The listing builds one solid part. Answer for the finished solid, in the listing's coordinates (mm). Round coordinates to 2 decimals unless told otherwise and drop trailing zeros. Loops run counter-clockwise (first coordinate to the right, second up) from the corner with the lowest first, then second, coordinate; pieces in that order, holes last. Notation, with made-up numbers: (-1, 83.5) -> (21, 83.5) arc R15 cw to (21, 99.5) -> close; hole circle Ø10 at (-29.5, 75.25). An arc over 180 degrees is marked (long way). Write each question's results on one line, items separated by ' | '. Start each with the question number.
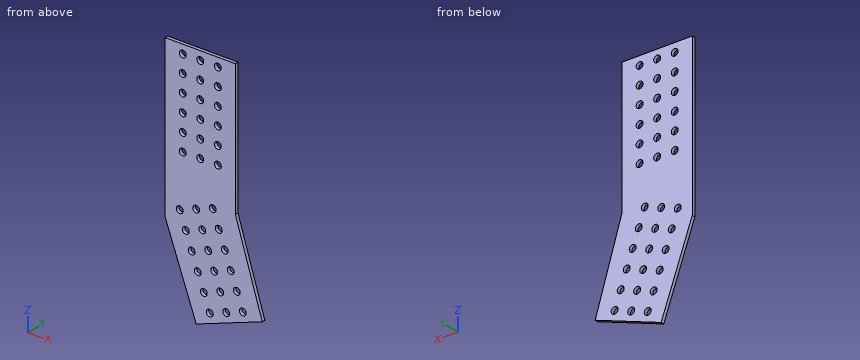
from build123d import *

# Parameters (mm, degrees)
SKETCH1_W           = 50.8
SKETCH1_H           = 76.2
SKETCH1_R           = 2.4892
BOSS_EXTRUDE1_DEPTH = 2.38125


with BuildPart() as part:
    # Sketch1 → Boss-Extrude1 (new body)
    # profile 1 of 3: a face of its own
    with BuildSketch(Plane(origin=(0, 0, 0), x_dir=(1, 0, 0), z_dir=(0, 1, 0))):
        with Locations((-99.145518613, -345.905622456)):
            Rectangle(SKETCH1_W, SKETCH1_H)
        with Locations(Location((-86.445518613, -326.855622456, 0), (0, 0, 90))):
            Circle(SKETCH1_R, mode=Mode.SUBTRACT)
        with Locations(Location((-86.445518613, -352.255622456, 0), (0, 0, 90))):
            Circle(SKETCH1_R, mode=Mode.SUBTRACT)
        with Locations(Location((-86.445518613, -377.655622456, 0), (0, 0, 90))):
            Circle(SKETCH1_R, mode=Mode.SUBTRACT)
        with Locations(Location((-99.145518613, -326.855622456, 0), (0, 0, 90))):
            Circle(SKETCH1_R, mode=Mode.SUBTRACT)
        with Locations(Location((-99.145518613, -352.255622456, 0), (0, 0, 90))):
            Circle(SKETCH1_R, mode=Mode.SUBTRACT)
        with Locations(Location((-99.145518613, -377.655622456, 0), (0, 0, 90))):
            Circle(SKETCH1_R, mode=Mode.SUBTRACT)
        with Locations(Location((-111.845518613, -377.655622456, 0), (0, 0, 90))):
            Circle(SKETCH1_R, mode=Mode.SUBTRACT)
        with Locations(Location((-111.845518613, -364.955622456, 0), (0, 0, 90))):
            Circle(SKETCH1_R, mode=Mode.SUBTRACT)
        with Locations(Location((-111.845518613, -352.255622456, 0), (0, 0, 90))):
            Circle(SKETCH1_R, mode=Mode.SUBTRACT)
        with Locations(Location((-111.845518613, -339.555622456, 0), (0, 0, 90))):
            Circle(SKETCH1_R, mode=Mode.SUBTRACT)
        with Locations(Location((-111.845518613, -326.855622456, 0), (0, 0, 90))):
            Circle(SKETCH1_R, mode=Mode.SUBTRACT)
        with Locations(Location((-111.845518613, -314.155622456, 0), (0, 0, 90))):
            Circle(SKETCH1_R, mode=Mode.SUBTRACT)
        with Locations(Location((-99.145518613, -364.955622456, 0), (0, 0, 90))):
            Circle(SKETCH1_R, mode=Mode.SUBTRACT)
        with Locations(Location((-99.145518613, -339.555622456, 0), (0, 0, 90))):
            Circle(SKETCH1_R, mode=Mode.SUBTRACT)
        with Locations(Location((-99.145518613, -314.155622456, 0), (0, 0, 90))):
            Circle(SKETCH1_R, mode=Mode.SUBTRACT)
        with Locations(Location((-86.445518613, -364.955622456, 0), (0, 0, 90))):
            Circle(SKETCH1_R, mode=Mode.SUBTRACT)
        with Locations(Location((-86.445518613, -339.555622456, 0), (0, 0, 90))):
            Circle(SKETCH1_R, mode=Mode.SUBTRACT)
        with Locations(Location((-86.445518613, -314.155622456, 0), (0, 0, 90))):
            Circle(SKETCH1_R, mode=Mode.SUBTRACT)
    # profile 2 of 3: a face of its own
    with BuildSketch(Plane(origin=(0, 0, 0), x_dir=(1, 0, 0), z_dir=(0, 1, 0))):
        Polygon((-73.745518613, -307.805622456), (-124.545518613, -307.805622456), (-124.545518613, -267.92136832), (-73.745518613, -286.411056221), align=None)
        with Locations(Location((-102.075911776, -280.451262674, 0), (0, 0, 90))):
            Circle(SKETCH1_R, mode=Mode.SUBTRACT)
        with Locations(Location((-114.01000806, -276.107606853, 0), (0, 0, 90))):
            Circle(SKETCH1_R, mode=Mode.SUBTRACT)
        with Locations(Location((-90.141815492, -284.794918494, 0), (0, 0, 90))):
            Circle(SKETCH1_R, mode=Mode.SUBTRACT)
    # profile 3 of 3: a face of its own
    with BuildSketch(Plane(origin=(0, 0, 0), x_dir=(1, 0, 0), z_dir=(0, 1, 0))):
        Polygon((-124.545518613, -267.92136832), (-73.745518613, -286.411056221), (-54.317612196, -223.501044752), (-102.053997332, -206.126421471), align=None)
        with Locations(Location((-72.767192211, -237.058533358, 0), (0, 0, 90))):
            Circle(SKETCH1_R, mode=Mode.SUBTRACT)
        with Locations(Location((-81.454503851, -260.926725926, 0), (0, 0, 90))):
            Circle(SKETCH1_R, mode=Mode.SUBTRACT)
        with Locations(Location((-80.357632674, -220.780781254, 0), (0, 0, 90))):
            Circle(SKETCH1_R, mode=Mode.SUBTRACT)
        with Locations(Location((-89.044944315, -244.648973822, 0), (0, 0, 90))):
            Circle(SKETCH1_R, mode=Mode.SUBTRACT)
        with Locations(Location((-97.732255955, -268.51716639, 0), (0, 0, 90))):
            Circle(SKETCH1_R, mode=Mode.SUBTRACT)
        with Locations(Location((-109.666352239, -264.173510569, 0), (0, 0, 90))):
            Circle(SKETCH1_R, mode=Mode.SUBTRACT)
        with Locations(Location((-105.322696419, -252.239414285, 0), (0, 0, 90))):
            Circle(SKETCH1_R, mode=Mode.SUBTRACT)
        with Locations(Location((-100.979040599, -240.305318001, 0), (0, 0, 90))):
            Circle(SKETCH1_R, mode=Mode.SUBTRACT)
        with Locations(Location((-96.635384779, -228.371221717, 0), (0, 0, 90))):
            Circle(SKETCH1_R, mode=Mode.SUBTRACT)
        with Locations(Location((-92.291728958, -216.437125433, 0), (0, 0, 90))):
            Circle(SKETCH1_R, mode=Mode.SUBTRACT)
        with Locations(Location((-93.388600135, -256.583070106, 0), (0, 0, 90))):
            Circle(SKETCH1_R, mode=Mode.SUBTRACT)
        with Locations(Location((-84.701288495, -232.714877538, 0), (0, 0, 90))):
            Circle(SKETCH1_R, mode=Mode.SUBTRACT)
        with Locations(Location((-85.798159671, -272.86082221, 0), (0, 0, 90))):
            Circle(SKETCH1_R, mode=Mode.SUBTRACT)
        with Locations(Location((-77.110848031, -248.992629642, 0), (0, 0, 90))):
            Circle(SKETCH1_R, mode=Mode.SUBTRACT)
        with Locations(Location((-68.42353639, -225.124437074, 0), (0, 0, 90))):
            Circle(SKETCH1_R, mode=Mode.SUBTRACT)
    extrude(amount=BOSS_EXTRUDE1_DEPTH)


solid = part.part
Item 1: The part is cut by section A-A, the plane z = 332.5. Give the vertices of the cut face in (x, y).
Item 2: Straight lines are drawn through the part: L1, parallel to X at y = 0.6, z = 327; L2, parallel to Z at x = -90.5, y = 1.7; L3, parallel to X at y = 1.95, z = 227. For each, find the intervals that lie inside material, in ascending order. Write a range as [from, to].
Item 3: The part is cut by section C-C, the plane y = 1.4. Give the number of separate pieces and of enclosed holes in the cut face, plus the area to 3 significant figures.
Item 4: The part is cut by section B-B, the plane x = -60. Give the vertices of the cut face in (y, z), plus the area to 3 significant figures.
Item 5: This flat-tipped pin is pushed along its axis until it touches: pin 1 Ø3 at (x, z) = (-99.15, 326.86) entering from +Y. Where does it stop, or does it pass through?
Report:
1) outline: (-124.55, 0) -> (-73.75, 0) -> (-73.75, 2.38) -> (-124.55, 2.38) -> close
2) L1: x = [-124.55, -114.33], [-109.36, -101.63], [-96.66, -88.93], [-83.96, -73.75] | L2: z = [210.33, 214.71], [218.17, 242.63], [246.67, 282.33], [287.26, 384.01] | L3: x = [-109.65, -98.71], [-94.56, -70.06], [-66.79, -55.4]
3) separate pieces: 1 | enclosed holes: 36 | area: 8,170 mm2
4) outline: (0, 221.43) -> (2.38, 221.43) -> (2.38, 241.9) -> (0, 241.9) -> close | area: 48.7 mm2
5) pin 1: passes through
